```python
from build123d import *

# Parameters (mm, degrees)
BOSS_EXTRUDE1_DEPTH      = 3.5
FILLET1_R                = 15.875
SKETCH3_R                = 3.75
BOSS_EXTRUDE2_DEPTH      = 3
BOSS_EXTRUDE2_DEPTH_BACK = 9.99999997
CUT_EXTRUDE1_DEPTH       = 13.99999997


with BuildPart() as part:
    # Sketch1 → Boss-Extrude1 (new body, symmetric)
    with BuildSketch(Plane.XY):
        Polygon((1.5875, -1.5875), (1.5875, -33.4645), (-1.5875, -33.4645), (-1.5875, -1.5875), (-33.4645, -1.5875), (-33.4645, 1.5875), (-1.5875, 1.5875), (-1.5875, 33.4645), (1.5875, 33.4645), (1.5875, 1.5875), (33.4645, 1.5875), (33.4645, -1.5875), align=None)
    extrude(amount=BOSS_EXTRUDE1_DEPTH, both=True)

    # Fillet1
    fillet1_edges = [part.edges().sort_by_distance(p)[0] for p in [
        (-1.5875, 1.5875, 0),
        (1.5875, 1.5875, 0),
        (1.5875, -1.5875, 0),
        (-1.5875, -1.5875, 0),
    ]]
    fillet(fillet1_edges, radius=FILLET1_R)

    # Sketch3 → Boss-Extrude2 (add, two sides)
    with BuildSketch(Plane(origin=(0, 0, -3.5), x_dir=(-1, 0, 0), z_dir=(0, 0, -1))) as boss_extrude2_sk:
        Circle(SKETCH3_R)
    extrude(amount=BOSS_EXTRUDE2_DEPTH)
    extrude(boss_extrude2_sk.sketch, amount=-BOSS_EXTRUDE2_DEPTH_BACK)

    # Sketch4 → Cut-Extrude1 (cut, through all)
    with BuildSketch(Plane(origin=(0, 0, -6.5), x_dir=(-1, 0, 0), z_dir=(0, 0, -1))):
        with BuildLine():
            Line((-0.889, 0.8255), (-0.889, 2.4765))
            ThreePointArc((-0.889, 2.4765), (0, 2.633207345), (0.889, 2.4765))
            Line((0.889, 2.4765), (0.889, 0.8255))
            Line((0.889, 0.8255), (2.54, 0.8255))
            ThreePointArc((2.54, 0.8255), (2.674528493, 0), (2.54, -0.8255))
            Line((2.54, -0.8255), (0.889, -0.8255))
            Line((0.889, -0.8255), (0.889, -2.4765))
            ThreePointArc((0.889, -2.4765), (0, -2.633207345), (-0.889, -2.4765))
            Line((-0.889, -2.4765), (-0.889, -0.8255))
            Line((-0.889, -0.8255), (-2.54, -0.8255))
            ThreePointArc((-2.54, -0.8255), (-2.674528493, 0), (-2.54, 0.8255))
            Line((-2.54, 0.8255), (-0.889, 0.8255))
        make_face()
    extrude(amount=-CUT_EXTRUDE1_DEPTH, mode=Mode.SUBTRACT)


solid = part.part
```
Part model, mm, in its own coordinate system. A direction names the side the tool comes from. Give positions to 0.01 mm unless a question says otherwise; leave off trailing zeros. Loops run counter-clockwise (first coordinate to the right, second up) from the corner with the lowest first, then second, coordinate; pieces in that order, holes last. Notation, with made-up numbers: M 18,-12 L 72,-12 A36 cw 72,27 Z; hole C -36,46.25 d6. An arc over 180 degrees is marked long. Return JSON: item names as keys, results as strings.
1) 3-axis set-ups, long thin cutter, end or side, ignore diameter. For faces 1 (the face through (1.588, -25, 0)), 2 (the face through (2, 0.826, 0)), 3 (the face through (-5, 0, 3.5)), 4 (the face through (-1.588, -26, 0)): which of +Z, -Z, +X, -X, +Y, -Y reach the whole face in a straight line?
Calculated:
{"face 1": "+Z, -Z, +X, -Y", "face 2": "+Z, -Z", "face 3": "+Z", "face 4": "+Z, -Z, -X, -Y"}
2) Pull direction X, two halves, no side cores. Call faces 5 (the face through (-2, -0.826, 0)), 6 (the face through (-6.114, 6.361, -0.049)), 7 (the face through (3.746, 0.165, -4.979)): released by +X, released by -X, zero draft, split by the parting line, or undercut.
Calculated:
{"face 5": "undercut", "face 6": "released by -X", "face 7": "split by the parting line"}
3) Flat gauge pins, fed straight in: pin 1 Ø2 at (y, z) = (-21, 2.5) entering from +X; pin 2 Ø2 at (x, z) = (28.5, -1) entering from -Y; pin 3 Ø1 at (x, z) = (6.5, 2) entering from +Y; pin 4 Ø1.3 at (x, z) = (-2, -3) entering from -Y. Where does each tip first touch, or does it go through?
Calculated:
{"pin 1": "stops at x = 1.59", "pin 2": "stops at y = -1.59", "pin 3": "stops at y = 6.48", "pin 4": "stops at y = -33.46"}
4) Saw through at B-B, the plane y = 0. List the corners of the cut face in (x, z), then the cut area to 3 significant figures.
Calculated:
{"outline": "M -33.46,-3.5 L -3.75,-3.5 L -3.75,-6.5 L -2.67,-6.5 L -2.67,6.5 L -3.75,6.5 L -3.75,3.5 L -33.46,3.5 Z; M 2.67,-6.5 L 3.75,-6.5 L 3.75,-3.5 L 33.46,-3.5 L 33.46,3.5 L 3.75,3.5 L 3.75,6.5 L 2.67,6.5 Z", "area": "444 mm2"}
5) Saw through at A-A, the plane x = 0. List the corners of the cut face in (y, z).
Calculated:
{"outline": "M -33.46,-3.5 L -3.75,-3.5 L -3.75,-6.5 L -2.63,-6.5 L -2.63,6.5 L -3.75,6.5 L -3.75,3.5 L -33.46,3.5 Z; M 2.63,-6.5 L 3.75,-6.5 L 3.75,-3.5 L 33.46,-3.5 L 33.46,3.5 L 3.75,3.5 L 3.75,6.5 L 2.63,6.5 Z"}
6) Drill centre lines: line 1 (X direction, y = 18, z = -1); line 2 (Z direction, x = -2.5, y = 3.5). Where is each one in solid material? Low to high.
Calculated:
{"line 1": "x = -1.59 to 1.59", "line 2": "z = -3.5 to 3.5"}
7) Saw through at D-D, the plane x = -19. List the corners of the cut face in (y, z), then the cut area to 3 significant figures.
Calculated:
{"outline": "M -1.59,-3.5 L 1.59,-3.5 L 1.59,3.5 L -1.59,3.5 Z", "area": "22.2 mm2"}
